Model file for the job. Use its own axes, mm. Face numbers are marked on the shaded views. A direction names the side the tool comes from. Round coordinates to 2 decimals unless told otherwise and drop trailing zeros. Loops run counter-clockwise (first coordinate to the right, second up) from the corner with the lowest first, then second, coordinate; pieces in that order, holes last. Notation, with made-up numbers: M 32.5,75 L 64.5,75 A36 cw 64.5,110 Z; hole C 78.25,8 d6. An arc over 180 degrees is marked long. Use a Markdown table: item, result. Add a question column.
Item 1: Saw through at D-D on x = -0.5. Write the cut outline in (y, z) (3 decimals).
Item 2: Saw through at A-A on x = 1. Write the cut outline in (y, z) (3 decimals).
Item 3: Saw through at C-C on z = 21. Write the cut outline in (x, y).
Item 4: Pin check, flat tips, straight feed: P1, Ø1.5, axis at x = 2.5, z = 23.5, coming from the +Y side; P2, Ø2, axis at x = 1, z = 1.5, coming from the +Y side. Stop position of each tip, or through.
Item 5: Saw through at B-B on y = -8. Write the cut outline in (x, z) (3 decimals), then the cut area to 3 significant figures.
Item 6: Tool access for the marked faces 1 and 2: list every direction of +Z, -Z, +X, -X, +Y, -Y with a clear straight run to the whole face (end or side of a thin tool).
Item 7: Wall check: L1, parallel to Z at x = 1, y = -10.75 (3 decimals); L2, parallel to Z at x = -2.75, y = -11 (3 decimals); L3, parallel to Y at x = -2, z = -0.5. Give the ranges that are in metal, low to high. Write a range as from..to.
```python
from build123d import *

# Parameters (mm, degrees)
F1_R     = 1.5812951981
F2_DEPTH = 34.925
F0_R     = 3.175
F3_DEPTH = 3.175
F5_DEPTH = 2.0052631579


# Not quite as in the source:
# - a length typed as a fraction of an inch, garbled in the dataset ("3 / 203.2 mm" for 3/8 in), is restored


with BuildPart() as f2:
    # F1 (on face) → F2 (new body)
    with BuildSketch(Plane.XY):
        with Locations((-0.0677817225, -10.2201197296)):
            Circle(F1_R)
    extrude(amount=F2_DEPTH)

    # F0 (on Top) → F3 (join)
    with BuildSketch(Plane.XY):
        with Locations((-0.0676529453, -10.2237053216)):
            Circle(F0_R)
    extrude(amount=-F3_DEPTH)

    # F4 (on face) → F5 (cut)
    with BuildSketch(Plane(origin=(0, 0, -3.175), x_dir=(1, 0, 0), z_dir=(0, 0, -1))):
        Polygon((-0.0660723406, 12.0567917448), (-1.6543620528, 11.141617377), (-1.6559426575, 9.3085309538), (-0.06923355, 8.3906188983), (1.5190561622, 9.3057932661), (1.5206367669, 11.1388796893), align=None)
    extrude(amount=-F5_DEPTH, mode=Mode.SUBTRACT)


solid = f2.part
```
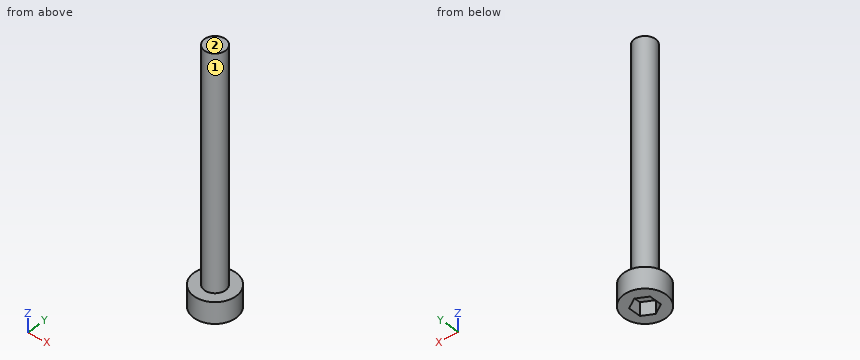
Entries:
| question | item | result |
|---|---|---|
| 1 | outline | M -13.369,-3.175 L -11.807,-3.175 L -11.807,-1.17 L -8.64,-1.17 L -8.64,-3.175 L -7.078,-3.175 L -7.078,0 L -8.699,0 L -8.699,34.925 L -11.741,34.925 L -11.741,0 L -13.369,0 Z |
| 2 | outline | M -13.214,-3.175 L -11.44,-3.175 L -11.44,-1.17 L -9.007,-1.17 L -9.007,-3.175 L -7.234,-3.175 L -7.234,0 L -9.054,0 L -9.054,34.925 L -11.386,34.925 L -11.386,0 L -13.214,0 Z |
| 3 | outline | C -0.07,-10.22 d3.16 |
| 4 | P1 | through |
| 4 | P2 | y = -8.64 |
| 5 | outline | M -2.334,-3.175 L 2.199,-3.175 L 2.199,0 L -2.334,0 Z |
| 5 | area | 14.4 mm2 |
| 6 | face 1 | +Z |
| 6 | face 2 | +Z, +X, -X, +Y, -Y |
| 7 | L1 | -1.17..34.925 |
| 7 | L2 | -3.175..0 |
| 7 | L3 | -12.74..-7.7 |
